Can you work these out from the drawing? Everything is in mm from the part's minimum corner. A direction names the side the tool comes from. Coordinates: 2 decimals unless noted, no trailing zeros. Loops run counter-clockwise (first coordinate to the right, second up) from the corner with the lowest first, then second, coordinate; pieces in that order, holes last.
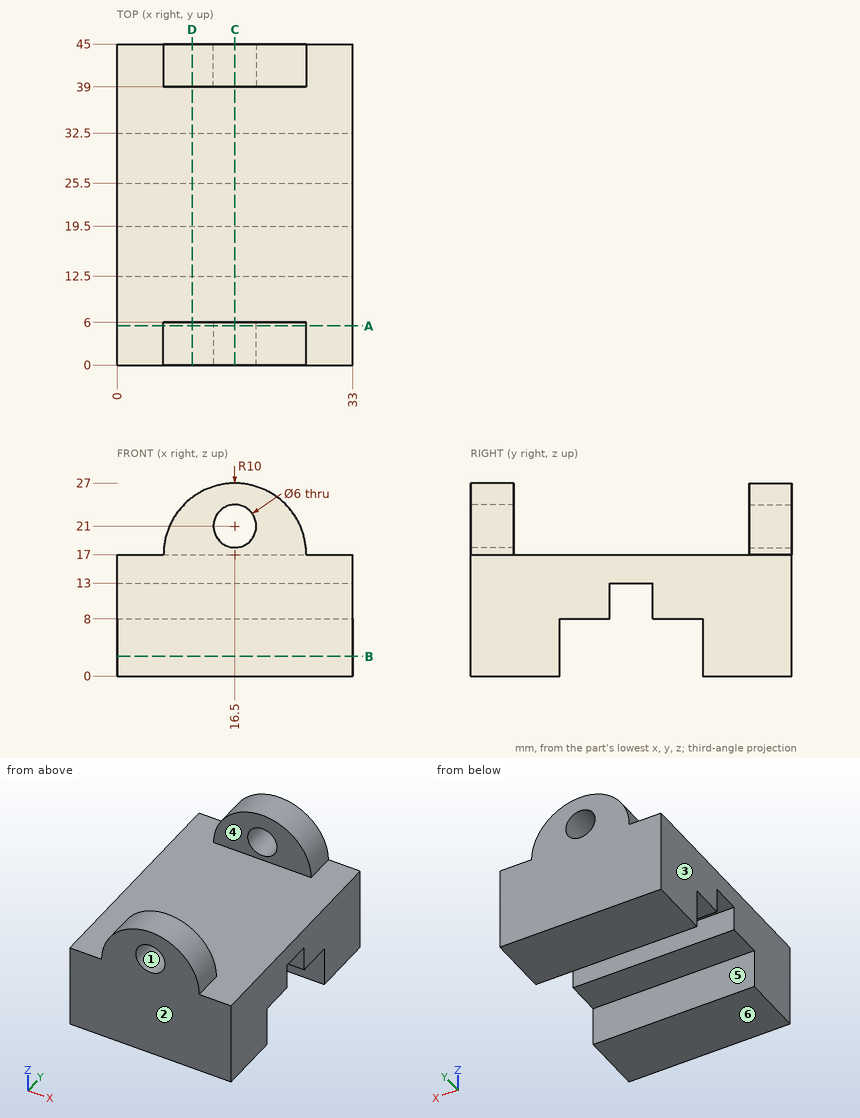
(1) Imagine slicing it at C-C, the plane x = 16.5. Write out the boundary of the cut face in (y, z), and give its area (3 significant figures).
Answers:
outline: (0, 0) - (12.5, 0) - (12.5, 8) - (19.5, 8) - (19.5, 13) - (25.5, 13) - (25.5, 8) - (32.5, 8) - (32.5, 0) - (45, 0) - (45, 18) - (39, 18) - (39, 17) - (6, 17) - (6, 18) - (0, 18) - close; (0, 24) - (6, 24) - (6, 27) - (0, 27) - close; (39, 24) - (45, 24) - (45, 27) - (39, 27) - close
area: 623 mm2
(2) Which directions (+Z, -Z, +X, -X, +Y, -Y) give clear straight access to the entire face, cutting with the end or side of a thin tool? Please do the marked faces 4, 5 and 6.
Answers:
face 4: +Z, +X, -X
face 5: -Z, +X, -X
face 6: -Z, +X, -X, +Y, -Y
(3) I need wall thicknesses on probe 1 along Y at (x, z) = (3.5, 10.75); probe 2 along Y at (x, z) = (9, 17.5); probe 3 along Z at (x, y) = (16, 4). Which ranges of each line are inside material? Lowest first, please.
Answers:
probe 1: y = 0 to 19.5, 25.5 to 45
probe 2: y = 0 to 6, 39 to 45
probe 3: z = 0 to 18.04, 23.96 to 26.99
(4) Imagine slicing it at B-B, the plane z = 2.75. Write out the boundary of the cut face in (x, y), and give its area (3 significant figures).
Answers:
outline: (0, 0) - (33, 0) - (33, 12.5) - (0, 12.5) - close; (0, 32.5) - (33, 32.5) - (33, 45) - (0, 45) - close
area: 825 mm2
(5) Imagine slicing it at D-D, the plane x = 10.5. Write out the boundary of the cut face in (y, z), and give its area (3 significant figures).
Answers:
outline: (0, 0) - (12.5, 0) - (12.5, 8) - (19.5, 8) - (19.5, 13) - (25.5, 13) - (25.5, 8) - (32.5, 8) - (32.5, 0) - (45, 0) - (45, 25) - (39, 25) - (39, 17) - (6, 17) - (6, 25) - (0, 25) - close
area: 671 mm2
(6) For pin 1 (3.5 mm diameter, centred on x = 8.5, y = 28.5, fed in from -Z); pin 2 (4 mm diameter, centred on y = 7.5, z = 21, fed in from -X) (3 decimals); pin 3 (1.5 mm diameter, centred on x = 23.5, y = 25, fed in from +Z), each with a flat end and sliding along its axis, tell me the tip position at first contact or that it passes through.
Answers:
pin 1: stops at z = 8
pin 2: stops at x = 6.865
pin 3: stops at z = 17
(7) We'd pull the mould along X, two halves only. Please class the marked faces 1, 2 and 3: +X half, -X half, draft (parallel to the pull), parting line (faces both ways), or undercut.
Answers:
face 1: undercut
face 2: draft
face 3: -X half
(8) Imagine slicing it at A-A, the plane y = 5.5. Write out the boundary of the cut face in (x, z).
Answers:
outline: (0, 0) - (33, 0) - (33, 17) - (26.5, 17) arc R10 ccw to (6.5, 17) - (0, 17) - close; hole circle Ø6 at (16.5, 21)
